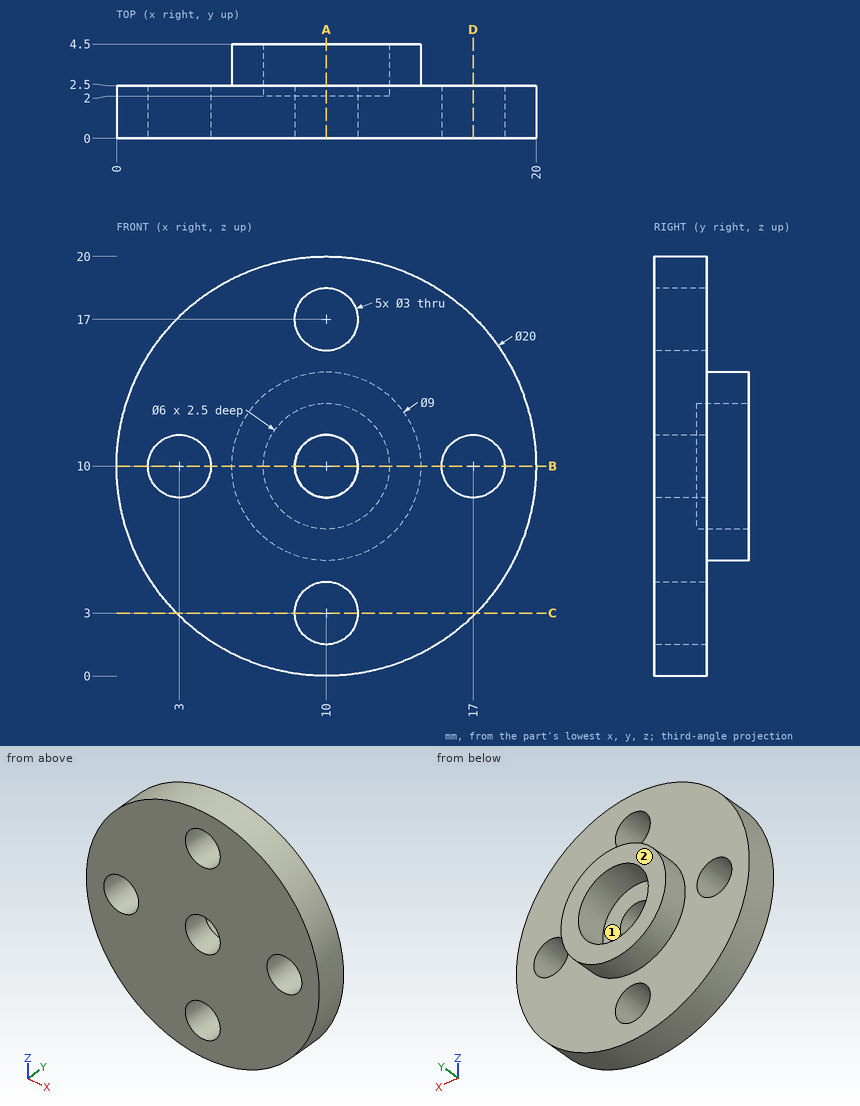
Can you work these out from the drawing? Everything is in mm from the part's minimum corner. A direction names the side the tool comes from. Round coordinates to 2 decimals unless told otherwise and drop trailing zeros. Loops run counter-clockwise (first coordinate to the right, second up) from the corner with the lowest first, then second, coordinate; pieces in that order, holes last. Notation, with made-up numbers: (70, -2) - (112, -2) arc R9 ccw to (112, 9) - close; hole circle Ø11 at (37, 28.5). An arc over 180 degrees is marked (long way). Answer in a Markdown table with one row per item. Add a question column.
(1) I'm going to push flat-ended pins straight in: pin 1 (1.5 mm diameter, centred on x = 13, z = 4.5, fed in from +Y); pin 2 (1.8 mm diameter, centred on x = 10, z = 10, fed in from +Y); pin 3 (5 mm diameter, centred on x = 10, z = 10, fed in from +Y). Where does each tip first touch, or does it pass through?
(2) If we section it at D-D (x = 17): Please give me the cut outline in (y, z), plus the area to 3 significant figures.
(3) I need wall thicknesses on line 1 along X through (y, z) = (1.4, 10); line 2 along Y through (x, z) = (11.75, 10.5); line 3 along Y through (x, z) = (18.5, 5.75). Which ranges of each line are inside material? Lowest first, please.
(4) If we section it at A-A (x = 10): Please give me the cut outline in (y, z).
(5) For the marked faces 1 and 2, which set-ups out of +Z, -Z, +X, -X, +Y, -Y let a thin tool reach every point of the face, with its end or its side?
(6) If we section it at C-C (z = 3): Please give me the cut outline in (x, y).
(7) If we section it at B-B (z = 10): Please give me the cut outline in (x, y).
Model answer:
| question | item | result |
|---|---|---|
| 1 | pin 1 | stops at y = 2.5 |
| 1 | pin 2 | passes through |
| 1 | pin 3 | stops at y = 2 |
| 2 | outline | (0, 2.86) - (2.5, 2.86) - (2.5, 8.5) - (0, 8.5) - close; (0, 11.5) - (2.5, 11.5) - (2.5, 17.14) - (0, 17.14) - close |
| 2 | area | 28.2 mm² |
| 3 | line 1 | x = 0 to 1.5, 4.5 to 8.5, 11.5 to 15.5, 18.5 to 20 |
| 3 | line 2 | y = 0 to 2 |
| 3 | line 3 | y = 0 to 2.5 |
| 4 | outline | (0, 0) - (2.5, 0) - (2.5, 1.5) - (0, 1.5) - close; (0, 4.5) - (2.5, 4.5) - (2.5, 5.5) - (4.5, 5.5) - (4.5, 7) - (2, 7) - (2, 8.5) - (0, 8.5) - close; (0, 11.5) - (2, 11.5) - (2, 13) - (4.5, 13) - (4.5, 14.5) - (2.5, 14.5) - (2.5, 15.5) - (0, 15.5) - close; (0, 18.5) - (2.5, 18.5) - (2.5, 20) - (0, 20) - close |
| 5 | face 1 | +Y |
| 5 | face 2 | +Z, -Z, +X, -X, +Y |
| 6 | outline | (2.86, 0) - (8.5, 0) - (8.5, 2.5) - (2.86, 2.5) - close; (11.5, 0) - (17.14, 0) - (17.14, 2.5) - (11.5, 2.5) - close |
| 7 | outline | (0, 0) - (1.5, 0) - (1.5, 2.5) - (0, 2.5) - close; (4.5, 0) - (8.5, 0) - (8.5, 2) - (7, 2) - (7, 4.5) - (5.5, 4.5) - (5.5, 2.5) - (4.5, 2.5) - close; (11.5, 0) - (15.5, 0) - (15.5, 2.5) - (14.5, 2.5) - (14.5, 4.5) - (13, 4.5) - (13, 2) - (11.5, 2) - close; (18.5, 0) - (20, 0) - (20, 2.5) - (18.5, 2.5) - close |
